Here's the drawing with two shaded views (mm, measured from the low corner). I have some questions. Coordinates: 2 decimals unless noted, no trailing zeros. Loops run counter-clockwise (first coordinate to the right, second up) from the corner with the lowest first, then second, coordinate; pieces in that order, holes last. Notation, with made-up numbers: (-19.75, -20.5) -> (22.25, -20.5) arc R16 cw to (22.25, 2.5) -> close; hole circle Ø10 at (-12.5, 44). An arc over 180 degrees is marked (long way). Answer as a JSON object with one key per item and string values. Group by question number.
Q1. I want a section at C-C on z = 4. Write out the boundary of the cut face in (x, y).
Q2. I want a section at B-B on x = 8. Write out the boundary of the cut face in (y, z), then the cut area to 3 significant figures.
Q3. I want a section at D-D on x = 5. Write out the boundary of the cut face in (y, z).
Q4. I need wall thicknesses on line 1 (Y direction, x = 8, z = 7.5); line 2 (Y direction, x = 7.25, z = 2.75); line 3 (Y direction, x = 12, z = 0.75). Which ranges of each line are inside material? Lowest first, please.
Q5. I'm going to push flat-ended pins straight in: pin 1 (1 mm diameter, centred on x = 8, z = 2, fed in from -Y); pin 2 (3 mm diameter, centred on x = 8, y = 32.5, fed in from -Z). Where does each tip first touch, or does it pass through?
Q6. I want a section at A-A on y = 20. Write out the boundary of the cut face in (x, z), then the cut area to 3 significant figures.
Q7. Thinking about a two-plate mould opening in Y: for the marked faces 1, 2, 3 and 4, which applies, released by +Y, released by -Y, zero draft, split by the parting line, or undercut?
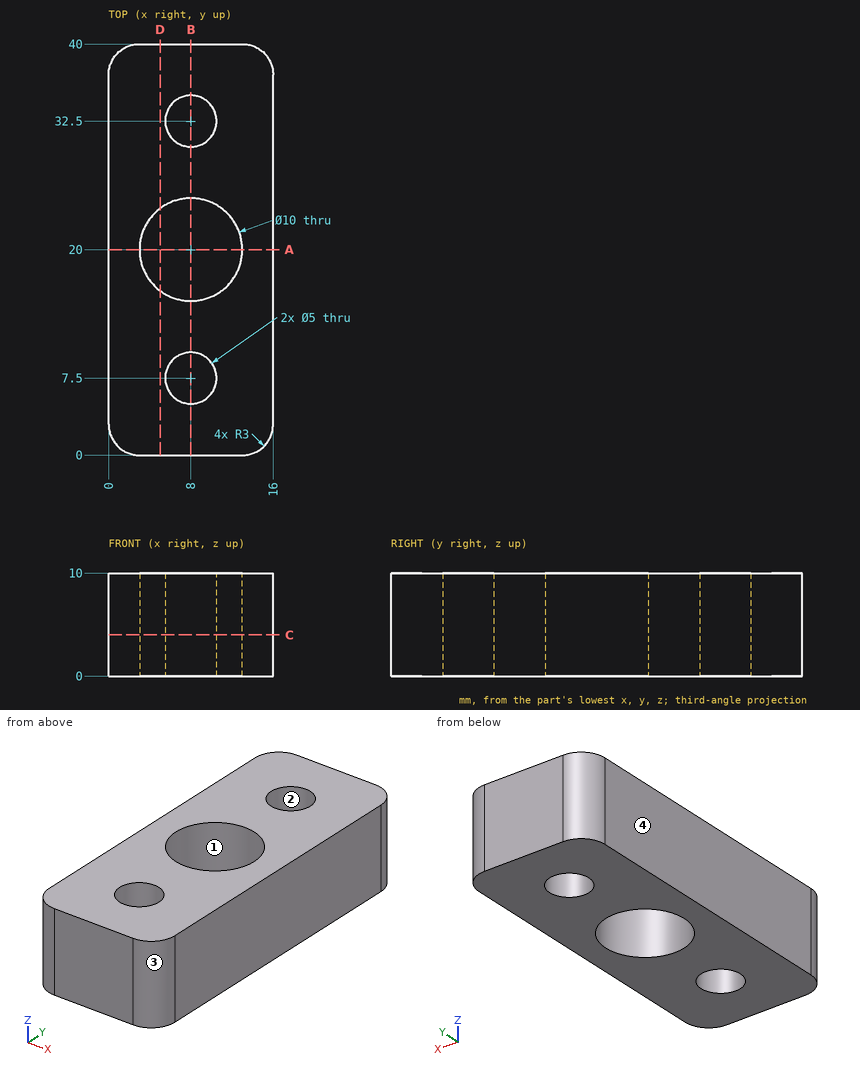
Result set:
{
 "1": {"outline": "(0, 3) arc R3 ccw to (3, 0) -> (13, 0) arc R3 ccw to (16, 3) -> (16, 37) arc R3 ccw to (13, 40) -> (3, 40) arc R3 ccw to (0, 37) -> close; hole circle Ø10 at (8, 20); hole circle Ø5 at (8, 7.5); hole circle Ø5 at (8, 32.5)"},
 "2": {"outline": "(0, 0) -> (5, 0) -> (5, 10) -> (0, 10) -> close; (10, 0) -> (15, 0) -> (15, 10) -> (10, 10) -> close; (25, 0) -> (30, 0) -> (30, 10) -> (25, 10) -> close; (35, 0) -> (40, 0) -> (40, 10) -> (35, 10) -> close", "area": "200 mm²"},
 "3": {"outline": "(0, 0) -> (16, 0) -> (16, 10) -> (0, 10) -> close; (24, 0) -> (40, 0) -> (40, 10) -> (24, 10) -> close"},
 "4": {"line 1": "y = 0 to 5, 10 to 15, 25 to 30, 35 to 40", "line 2": "y = 0 to 5.12, 9.88 to 15.06, 24.94 to 30.12, 34.88 to 40", "line 3": "y = 0 to 17, 23 to 40"},
 "5": {"pin 1": "stops at y = 0", "pin 2": "passes through"},
 "6": {"outline": "(0, 0) -> (3, 0) -> (3, 10) -> (0, 10) -> close; (13, 0) -> (16, 0) -> (16, 10) -> (13, 10) -> close", "area": "60.0 mm²"},
 "7": {"face 1": "undercut", "face 2": "undercut", "face 3": "released by -Y", "face 4": "zero draft"}
}
